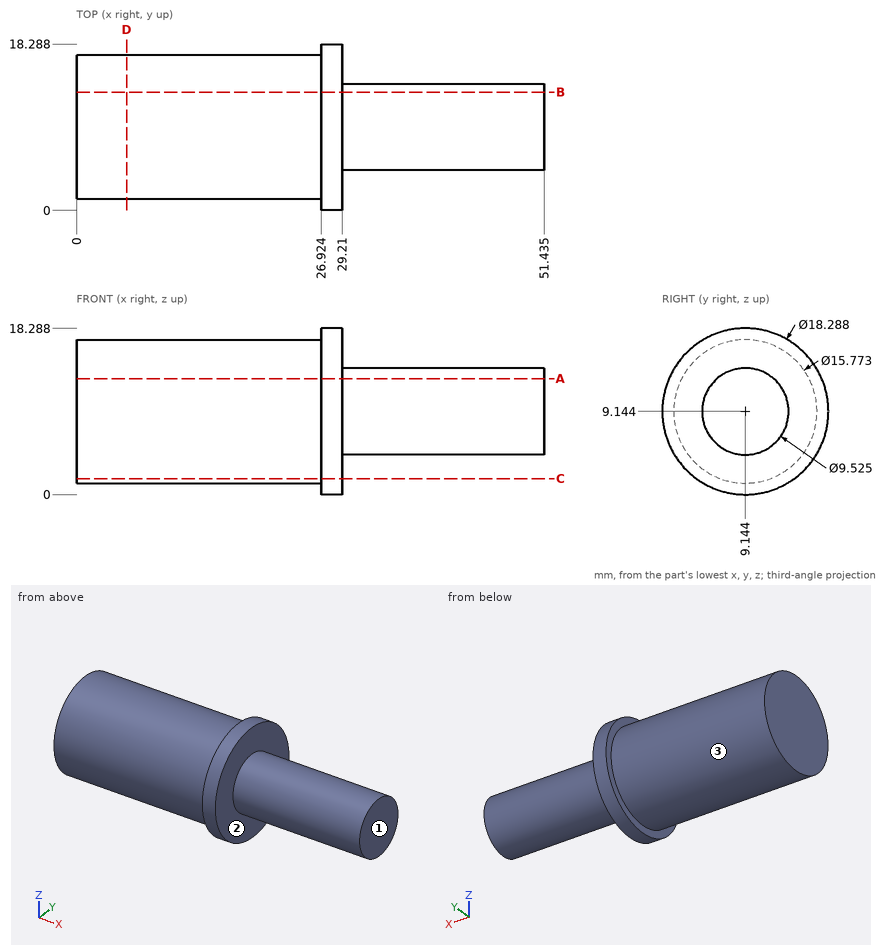
For this review, use the dimensioned drawing (mm, ordinates from the lowest corner) and the shaded views. A direction names the side the tool comes from. Coordinates: 2 decimals unless noted, no trailing zeros. Loops run counter-clockwise (first coordinate to the right, second up) from the corner with the lowest first, then second, coordinate; pieces in that order, holes last. Notation, with made-up numbers: (0, -35) -> (15, -35) arc R18 ccw to (15, -5) -> close; hole circle Ø2 at (1.5, 20.25). An arc over 180 degrees is marked (long way). Return JSON: item names as keys, results as strings. Group by question number.
(1) For pin 1 Ø3 at (x, z) = (9, 6) entering from +Y; pin 2 Ø6 at (x, z) = (8.5, 3) entering from +Y; pin 3 Ø3 at (x, z) = (44.5, 9) entering from +Y, all flat-tipped, find the tip position at first contact; note any pin that passes through.
(2) To check wall thickness, follow L1, parallel to Z at x = 3.5, y = 9.5 (1 decimal); L2, parallel to Y at x = 19.5, z = 9.25; L3, parallel to Z at x = 27, y = 8.75. State the ranges of each line that lie inside material, in increasing order.
(3) Tool access review of the marked faces 1, 2 and 3: name each direction out of +Z, -Z, +X, -X, +Y, -Y from which nothing blocks a thin tool from reaching the whole face with its end or side.
(4) Consider section B-B, the plane y = 13. Give the boundary of the cut face in (x, z) (1 decimal).
(5) Consider section D-D, the plane x = 5.5. Give the boundary of the cut face in (y, z), plus the area to 3 significant figures.
(6) Consider section C-C, the plane z = 1.75. Give the boundary of the cut face in (x, y) (1 decimal).
(7) Consider section A-A, the plane z = 12.75. Give the boundary of the cut face in (x, y) (1 decimal).
Results below:
{
 "1": {"pin 1": "stops at y = 16.86", "pin 2": "stops at y = 16.38", "pin 3": "stops at y = 13.91"},
 "2": {"L1": "z = 1.3 to 17", "L2": "y = 1.26 to 17.03", "L3": "z = 0.01 to 18.28"},
 "3": {"face 1": "+Z, -Z, +X, +Y, -Y", "face 2": "+X", "face 3": "-X"},
 "4": {"outline": "(0, 2.3) -> (26.9, 2.3) -> (26.9, 0.9) -> (29.2, 0.9) -> (29.2, 6.3) -> (51.4, 6.3) -> (51.4, 11.9) -> (29.2, 11.9) -> (29.2, 17.4) -> (26.9, 17.4) -> (26.9, 16) -> (0, 16) -> close"},
 "5": {"outline": "circle Ø15.77 at (9.14, 9.14)", "area": "195 mm2"},
 "6": {"outline": "(0, 6.4) -> (26.9, 6.4) -> (26.9, 3.8) -> (29.2, 3.8) -> (29.2, 14.5) -> (26.9, 14.5) -> (26.9, 11.9) -> (0, 11.9) -> close"},
 "7": {"outline": "(0, 2.1) -> (26.9, 2.1) -> (26.9, 0.7) -> (29.2, 0.7) -> (29.2, 6) -> (51.4, 6) -> (51.4, 12.3) -> (29.2, 12.3) -> (29.2, 17.5) -> (26.9, 17.5) -> (26.9, 16.2) -> (0, 16.2) -> close"}
}
